Check sheet for the modelled part. Datum: model origin and axes. Units: mm. Face numbers are marked on the shaded views. A direction names the side the tool comes from. Round coordinates to 2 decimals unless told otherwise and drop trailing zeros. Order: outer loops, then holes, each group sorted by start corner. A loop starts at its lowest first (then second) coordinate and runs counter-clockwise, first axis right, second up.
Q1. Scan lines: probe 1 along Y at (x, z) = (0, 3.25); probe 2 along Y at (x, z) = (-31, 3.5); probe 3 along Z at (x, y) = (-20.5, 0). Record each from-to range of solid material in increasing order.
Q2. Mould release check, pull along Y, two halves, no side actions. Record for the marked faces 1, 2 and 3: +Y half, -Y half, draft (parallel to the pull), parting line (faces both ways), or undercut.
Q3. Depth check by flat-ended pin: P1, Ø5, axis at y = -24.5, z = 10.5, coming from the +X side; P2, Ø10, axis at x = 35.5, y = -37, coming from the -Z side; P3, Ø4, axis at x = -25.5, y = -2.5, coming from the +Z side. Enter the tip coordinate at first touch or a pass-through.
Q4. Cross-section at A-A on x = 0. Record the cut outline in (y, z), then the cut area to 3 significant figures.
Q5. Set-up check for the marked faces 4 and 5: record each of +Z, -Z, +X, -X, +Y, -Y from which the full face is reachable in a straight line by a thin tool's end or side.
from build123d import *

# Parameters (mm, degrees)
F0_R     = 47
F0_R_2   = 44
F1_DEPTH = 22.3
F0_R_3   = 41
F2_DEPTH = 10
F3_DEPTH = 5
F4_R     = 1
F5_SIZE  = 4.99999


# Not quite as in the source:
# - a fillet or chamfer is up to 0.001 mm smaller than in the source, because OpenCascade refuses the exact size


with BuildPart() as f1:
    # F0 (on Top) → F1 (new body)
    with BuildSketch(Plane.XY):
        Circle(F0_R)
        Circle(F0_R_2, mode=Mode.SUBTRACT)
    extrude(amount=F1_DEPTH)

    # F0 (on Top) → F2 (join)
    with BuildSketch(Plane.XY):
        Circle(F0_R_2)
        Circle(F0_R_3, mode=Mode.SUBTRACT)
    extrude(amount=F2_DEPTH)

    # F0 (on Top) → F3 (join)
    with BuildSketch(Plane.XY):
        Circle(F0_R)
        Circle(F0_R_2, mode=Mode.SUBTRACT)
        Circle(F0_R_2)
        Circle(F0_R_3, mode=Mode.SUBTRACT)
        Circle(F0_R_3)
    extrude(amount=-F3_DEPTH)

    # F4
    f4_edges = [f1.edges().sort_by_distance(p)[0] for p in [
        (-44, 0, 22.3),
        (-44, 0, 10),
        (-41, 0, 10),
        (-41, 0, 0),
    ]]
    fillet(f4_edges, radius=F4_R)

    # F5 (size 5 in the source; OpenCascade refuses exactly that, so slightly less here)
    f5_edges = [f1.edges().sort_by_distance(p)[0] for p in [
        (-47, 0, -5),
    ]]
    chamfer(f5_edges, length=F5_SIZE)


solid = f1.part
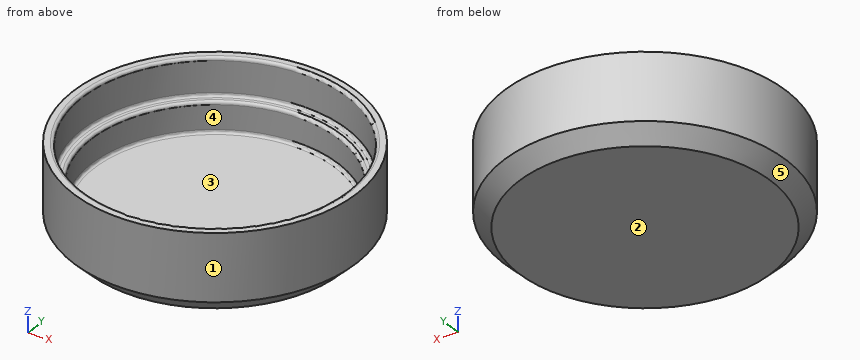
Results found:
1. probe 1: y = -47 to -41, 41 to 47
1. probe 2: y = -35.33 to -26.83, 26.83 to 35.33
1. probe 3: z = -5 to 0
2. face 1: parting line
2. face 2: draft
2. face 3: undercut
3. P1: stops at x = 41.53
3. P2: stops at z = -0.72
3. P3: stops at z = 0
4. outline: (-47, 0) - (-42, -5) - (42, -5) - (47, 0) - (47, 22.3) - (45, 22.3) arc R1 ccw to (44, 21.3) - (44, 11) arc R1 cw to (43, 10) - (42, 10) arc R1 ccw to (41, 9) - (41, 1) arc R1 cw to (40, 0) - (-40, 0) arc R1 cw to (-41, 1) - (-41, 9) arc R1 ccw to (-42, 10) - (-43, 10) arc R1 cw to (-44, 11) - (-44, 21.3) arc R1 ccw to (-45, 22.3) - (-47, 22.3) - close
4. area: 639 mm2
5. face 4: +Z
5. face 5: -Z
